Geometry: final body of the model. Coordinates: model frame, mm. Give positions to 0.01 mm unless a question says otherwise; leave off trailing zeros. Write each loop counter-clockwise with the first axis right and the second up, starting at its lowest first coordinate (ties: lowest second). Pieces come first, ordered by that corner, then holes.
Q1. Draft query along Z for faces 1 (the face through (-0.1, 8.5, 9)), 2 (the face through (-0.1, 8.5, -9)), 3 (the face through (9, 8.5, 0.1)), 4 (the face through (-3.955, 8.507, -4.658)). Return one class per face: pulls with the +Z half, pulls with the -Z half, needs draft (parallel to the pull), parting line crosses it, or undercut.
Q2. Cut plane C-C on y = 8.5. Return the cut outline in (x, z).
Q3. Cut plane B-B on z = 0.5. Return the cut outline in (x, y), plus the area to 3 significant figures.
Q4. Cut plane A-A on x = 1.75. Return the cut outline in (y, z), plus the area to 3 significant figures.
Q5. Line query: L1, parallel to X at y = 8.85, z = 0.5; L2, parallel to X at y = 8.6, z = -2; L3, parallel to Z at x = -2, y = 8.5. Output: solid intervals per line, ascending.
Q6. Pin query (flat end, axial travel): pin 1 (3 mm diameter, centred on x = 5.5, z = 0, fed in from +Y). Return the tip coordinate at first contact, or that it passes through.
```python
from build123d import *

# Parameters (mm, degrees)
SKETCH_1_W          = 18
SKETCH_1_H          = 18
EXTRUDE_1_DEPTH     = 8
CUT_EXTRUDE_START   = 8
SKETCH_5_W          = 16
SKETCH_5_H          = 17
CUT_EXTRUDE_6_DEPTH = 7
EXTRUDE_START       = 8
SKETCH_6_W          = 18
SKETCH_6_H          = 18
EXTRUDE_2_DEPTH     = 1
CUT_EXTRUDE_START_2 = 9
SKETCH_7_R          = 6.5
CUT_EXTRUDE_7_DEPTH = 1
SKETCH_11_W         = 18
SKETCH_11_H         = 18
CUT_EXTRUDE_9_DEPTH = 8


with BuildPart() as part:
    # 스케치1 → 보스-돌출1 (new body)
    with BuildSketch(Plane(origin=(0, 0, 0), x_dir=(1, 0, 0), z_dir=(0, 1, 0))):
        Rectangle(SKETCH_1_W, SKETCH_1_H)
    extrude(amount=EXTRUDE_1_DEPTH)

    # 스케치5 → 컷-돌출6 (cut)
    with BuildSketch(Plane(origin=(0, 0, 0), x_dir=(1, 0, 0), z_dir=(0, 1, 0)).offset(CUT_EXTRUDE_START)):
        with Locations((0, 0.5)):
            Rectangle(SKETCH_5_W, SKETCH_5_H)
    extrude(amount=-CUT_EXTRUDE_6_DEPTH, mode=Mode.SUBTRACT)

    # 스케치11 → 컷-돌출9 (cut)
    with BuildSketch(Plane.XZ):
        Rectangle(SKETCH_11_W, SKETCH_11_H)
    extrude(amount=-CUT_EXTRUDE_9_DEPTH, mode=Mode.SUBTRACT)


with BuildPart() as body_2:
    # 스케치6 → 보스-돌출2 (new body)
    with BuildSketch(Plane(origin=(0, 0, 0), x_dir=(1, 0, 0), z_dir=(0, 1, 0)).offset(EXTRUDE_START)):
        Rectangle(SKETCH_6_W, SKETCH_6_H)
    extrude(amount=EXTRUDE_2_DEPTH)

    # 스케치7 → 컷-돌출7 (cut)
    with BuildSketch(Plane(origin=(0, 0, 0), x_dir=(1, 0, 0), z_dir=(0, 1, 0)).offset(CUT_EXTRUDE_START_2)):
        with Locations(Location((0, -0.5, 0), (0, 0, 270))):
            Circle(SKETCH_7_R)
    extrude(amount=-CUT_EXTRUDE_7_DEPTH, mode=Mode.SUBTRACT)


solid = body_2.part
```
Data:
1. face 1: pulls with the +Z half
1. face 2: pulls with the -Z half
1. face 3: needs draft
1. face 4: undercut
2. outline: (-9, -9) - (9, -9) - (9, 9) - (-9, 9) - close; hole circle Ø13 at (0, 0.5)
3. outline: (-9, 8) - (-6.5, 8) - (-6.5, 9) - (-9, 9) - close; (6.5, 8) - (9, 8) - (9, 9) - (6.5, 9) - close
3. area: 5.00 mm2
4. outline: (8, -9) - (9, -9) - (9, -5.76) - (8, -5.76) - close; (8, 6.76) - (9, 6.76) - (9, 9) - (8, 9) - close
4. area: 5.48 mm2
5. L1: x = -9 to -6.5, 6.5 to 9
5. L2: x = -9 to -6, 6 to 9
5. L3: z = -9 to -5.68, 6.68 to 9
6. pin 1: stops at y = 9
